Can you work these out from the model? Positions are in its coordinate system, mm. A direction names the side the tool comes from. Give positions to 0.01 mm unless a question says otherwise; leave off trailing zeros. Loops run counter-clockwise (first coordinate to the right, second up) from the corner with the lowest first, then second, coordinate; pieces in that order, holes last. Notation, with made-up numbers: (-12.5, -31.75) - (17.5, -31.75) arc R19 cw to (17.5, -7.75) - close; hole circle Ø3 at (21, -28.5). An arc over 180 degrees is marked (long way). Answer as a JSON object with one key per item and string values. Group by question number.
Item 1: Suppose I cut it at B-B on z = 29.5. Write out the boundary of the cut face in (x, y) (3 decimals).
Item 2: Suppose I cut it at A-A on z = 5. Write out the boundary of the cut face in (x, y) (3 decimals), and give its area (3 significant figures).
Item 3: Suppose I cut it at C-C on x = 9.5. Write out the boundary of the cut face in (y, z).
Item 4: Will these pins go through, and if not, where does the flat tip stop? pin 1 (9.5 mm diameter, centred on x = 29, y = 36, fed in from +Z); pin 2 (5.5 mm diameter, centred on x = 26, z = 19, fed in from +Y); pin 3 (2.5 mm diameter, centred on x = -27.5, z = 17.5, fed in from +Y); pin 4 (6.5 mm diameter, centred on x = -27.5, y = 19.5, fed in from +Z).
Item 5: Which directions (+Z, -Z, +X, -X, +Y, -Y) give clear straight access to the entire face, cutting with the end or side of a thin tool? Please do faces 4 (the flat face through (0, 27, 7)), 5 (the cylindrical face through (30.648, 24.437, 5.127)), 6 (the flat face through (-28, 4, 20)).
Item 6: Thinking about a two-plate mould opening in Y: for faces 1 (the flat face through (-28, 4, 32)), 2 (the flat face through (-35, 11, 6)), 3 (the cylindrical face through (-24.352, 24.437, 5.127)), which applies, pulls with the +Y half, pulls with the -Y half, needs draft (parallel to the pull), parting line crosses it, or undercut?
Item 7: Suppose I cut it at D-D on y = 34.5. Write out the boundary of the cut face in (x, z) (3 decimals), and give its area (3 significant figures).
Item 8: Please list where these lines run through material, in increasing order: L1, parallel to X at y = 2.8, z = 17.5; L2, parallel to Y at x = 27, z = 6; L3, parallel to X at y = 5.55, z = 17.5 (3 decimals).
from build123d import *

# Parameters (mm, degrees)
SKETCH1_W                                        = 70
SKETCH1_H                                        = 35
BOSS_EXTRUDE1_DEPTH                              = 7
SKETCH2_W                                        = 70
SKETCH2_H                                        = 7
BOSS_EXTRUDE2_DEPTH                              = 35
FILLET1_R                                        = 5
CBORE_FOR_M5_HEX_HEAD_MACHINE_SCREW1_D           = 5.5
CBORE_FOR_M5_HEX_HEAD_MACHINE_SCREW1_CBORE_D     = 11.71
CBORE_FOR_M5_HEX_HEAD_MACHINE_SCREW1_CBORE_DEPTH = 3.8
CBORE_FOR_M4_HEX_HEAD_MACHINE_SCREW2_D           = 4.5
CBORE_FOR_M4_HEX_HEAD_MACHINE_SCREW2_CBORE_D     = 10.59
CBORE_FOR_M4_HEX_HEAD_MACHINE_SCREW2_CBORE_DEPTH = 3


with BuildPart() as part:
    # Sketch1 → Boss-Extrude1 (new body)
    with BuildSketch(Plane(origin=(0, 0, 0), x_dir=(1, 0, 0), z_dir=(0, 1, 0))):
        with Locations((0, -17.5)):
            Rectangle(SKETCH1_W, SKETCH1_H)
    extrude(amount=BOSS_EXTRUDE1_DEPTH)

    # Sketch2 → Boss-Extrude2 (add)
    with BuildSketch(Plane(origin=(0, 7, 0), x_dir=(1, 0, 0), z_dir=(0, 1, 0))):
        with Locations((0, -3.5)):
            Rectangle(SKETCH2_W, SKETCH2_H)
    extrude(amount=BOSS_EXTRUDE2_DEPTH)

    # Fillet1
    fillet1_edges = [part.edges().sort_by_distance(p)[0] for p in [
        (0, 7, 7),
    ]]
    fillet(fillet1_edges, radius=FILLET1_R)

    # CBORE for M5 Hex Head Machine Screw1 (through all)
    with Locations(Plane.XY.offset(7)):
        with Locations((-27.5, 34.5), (27.5, 34.5), (27.5, 19.5), (-27.5, 19.5)):
            CounterBoreHole(CBORE_FOR_M5_HEX_HEAD_MACHINE_SCREW1_D / 2, CBORE_FOR_M5_HEX_HEAD_MACHINE_SCREW1_CBORE_D / 2, CBORE_FOR_M5_HEX_HEAD_MACHINE_SCREW1_CBORE_DEPTH)

    # CBORE for M4 Hex Head Machine Screw2 (through all)
    with Locations(Plane(origin=(0, 7, 0), x_dir=(1, 0, 0), z_dir=(0, 1, 0))):
        with Locations((-27.5, -17.5), (-27.5, -29.5), (27.5, -17.5), (27.5, -29.5)):
            CounterBoreHole(CBORE_FOR_M4_HEX_HEAD_MACHINE_SCREW2_D / 2, CBORE_FOR_M4_HEX_HEAD_MACHINE_SCREW2_CBORE_D / 2, CBORE_FOR_M4_HEX_HEAD_MACHINE_SCREW2_CBORE_DEPTH)


solid = part.part
Worked out:
{
 "1": {"outline": "(-35, 0) - (-29.75, 0) - (-29.75, 4) - (-32.795, 4) - (-32.795, 7) - (-35, 7) - close; (-25.25, 0) - (25.25, 0) - (25.25, 4) - (22.205, 4) - (22.205, 7) - (-22.205, 7) - (-22.205, 4) - (-25.25, 4) - close; (29.75, 0) - (35, 0) - (35, 7) - (32.795, 7) - (32.795, 4) - (29.75, 4) - close"},
 "2": {"outline": "(-35, 0) - (35, 0) - (35, 42) - (-35, 42) - close; hole circle Ø11.71 at (-27.5, 19.5); hole circle Ø11.71 at (-27.5, 34.5); hole circle Ø11.71 at (27.5, 19.5); hole circle Ø11.71 at (27.5, 34.5)", "area": "2,510 mm2"},
 "3": {"outline": "(0, 0) - (42, 0) - (42, 7) - (12, 7) arc R5 cw to (7, 12) - (7, 35) - (0, 35) - close"},
 "4": {"pin 1": "stops at z = 7", "pin 2": "stops at y = 4", "pin 3": "passes through", "pin 4": "stops at z = 3.2"},
 "5": {"face 4": "+Z, +X, -X, +Y", "face 5": "+Z", "face 6": "+Y"},
 "6": {"face 1": "pulls with the +Y half", "face 2": "needs draft", "face 3": "undercut"},
 "7": {"outline": "(-35, 0) - (-30.25, 0) - (-30.25, 3.2) - (-33.355, 3.2) - (-33.355, 7) - (-35, 7) - close; (-24.75, 0) - (24.75, 0) - (24.75, 3.2) - (21.645, 3.2) - (21.645, 7) - (-21.645, 7) - (-21.645, 3.2) - (-24.75, 3.2) - close; (30.25, 0) - (35, 0) - (35, 7) - (33.355, 7) - (33.355, 3.2) - (30.25, 3.2) - close", "area": "366 mm2"},
 "8": {"L1": "x = -35 to -29.75, -25.25 to 25.25, 29.75 to 35", "L2": "y = 0 to 13.67, 25.33 to 28.67, 40.33 to 42", "L3": "x = -35 to -32.795, -22.205 to 22.205, 32.795 to 35"}
}
